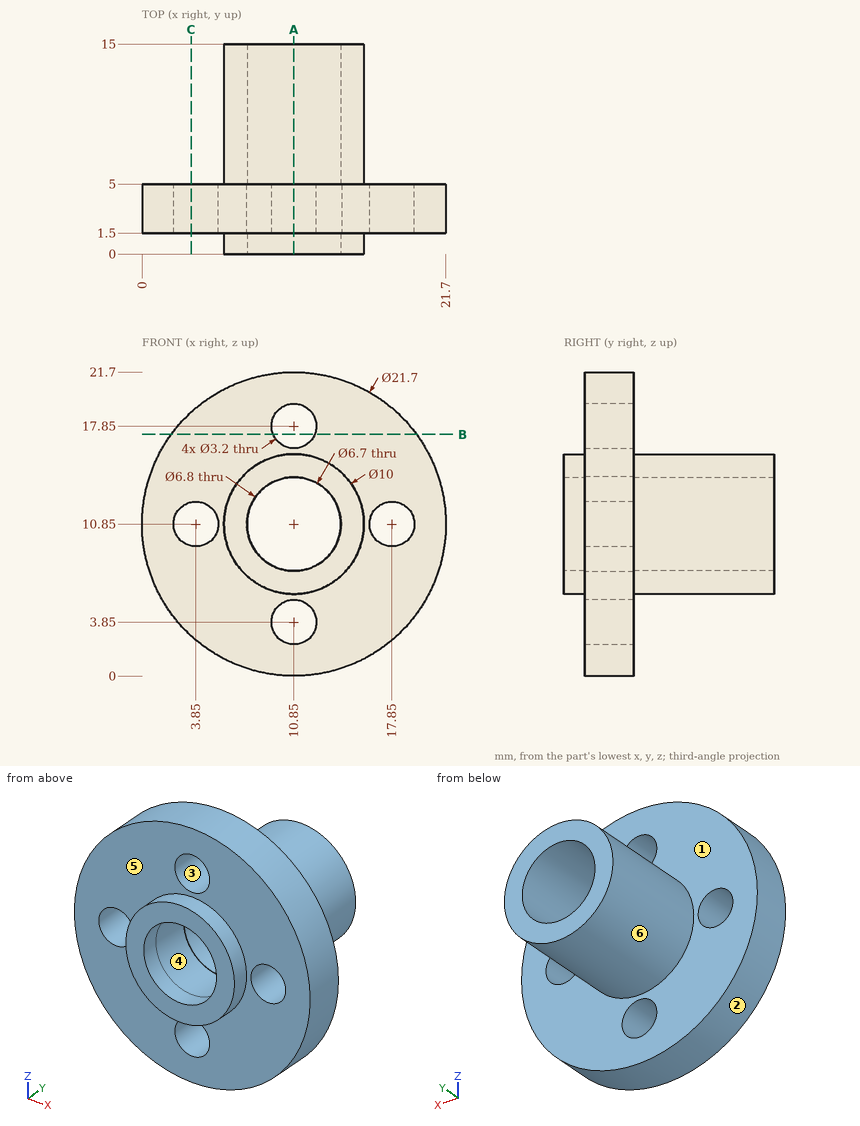
Geometry check sheet. Reference: drawing and pictorial views, mm from the part's lowest x, y, z. A direction names the side the tool comes from. Round coordinates to 2 decimals unless told otherwise and drop trailing zeros. Loops run counter-clockwise (first coordinate to the right, second up) from the corner with the lowest first, then second, coordinate; pieces in that order, holes last. Notation, with made-up numbers: (29, 39.25) - (63, 39.25) arc R19 ccw to (63, 52.25) - close; hole circle Ø4 at (-5, 69.5). An arc over 180 degrees is marked (long way). Use a Markdown table: item, result. Add a question column.
1. Section check A-A, the plane x = 10.85. Give the number of separate pieces and of enclosed holes in the cut face, plus the area to 3 significant figures.
2. Gauge pin test, flat ends, axial feed: pin 1 (8 mm diameter, centred on x = 15, z = 18, fed in from +Y); pin 2 (2 mm diameter, centred on y = 11, z = 7, fed in from +X); pin 3 (3 mm diameter, centred on y = 13, z = 13, fed in from +X); pin 4 (1.5 mm diameter, centred on x = 7, y = 1.5, fed in from -Z). Record the tip position at first contact, or that the pin passes through.
3. Section check B-B, the plane z = 17.25. Record the boundary of the cut face in (x, y), plus the area to 3 significant figures.
4. Access from +Z, -Z, +X, -X, +Y, -Y to the whole of each face (thin tool, end or side, straight path). Record for the marked faces 4, 5 and 6.
5. Section check C-C, the plane x = 3.5. Record the boundary of the cut face in (y, z), plus the area to 3 significant figures.
6. Thickness scan on probe 1 along X at (y, z) = (2.85, 10.85); probe 2 along Y at (x, z) = (17.75, 14.25); probe 3 along Z at (x, y) = (8.75, 12). Record the ranges inside material, lowest first. Write a range as [from, to].
7. Release check for a two-part mould opening along X. For the marked faces 1, 2 and 3 record: released by +X, released by -X, zero draft, split by the parting line, or undercut.
Checks:
| question | item | result |
|---|---|---|
| 1 | separate pieces | 4 |
| 1 | enclosed holes | 0 |
| 1 | area | 67.7 mm^2 |
| 2 | pin 1 | stops at y = 15 |
| 2 | pin 2 | stops at x = 14.96 |
| 2 | pin 3 | stops at x = 15.81 |
| 2 | pin 4 | stops at z = 0.45 |
| 3 | outline | (2.09, 1.5) - (9.37, 1.5) - (9.37, 5) - (2.09, 5) - close; (12.33, 1.5) - (19.61, 1.5) - (19.61, 5) - (12.33, 5) - close |
| 3 | area | 50.9 mm^2 |
| 4 | face 4 | none |
| 4 | face 5 | -Y |
| 4 | face 6 | +Y |
| 5 | outline | (1.5, 2.87) - (5, 2.87) - (5, 9.29) - (1.5, 9.29) - close; (1.5, 12.41) - (5, 12.41) - (5, 18.83) - (1.5, 18.83) - close |
| 5 | area | 44.9 mm^2 |
| 6 | probe 1 | x = [0, 2.25], [5.45, 7.45], [14.25, 16.25], [19.45, 21.7] |
| 6 | probe 2 | y = [1.5, 5] |
| 6 | probe 3 | z = [6.31, 8.24], [13.46, 15.39] |
| 7 | face 1 | zero draft |
| 7 | face 2 | split by the parting line |
| 7 | face 3 | undercut |
